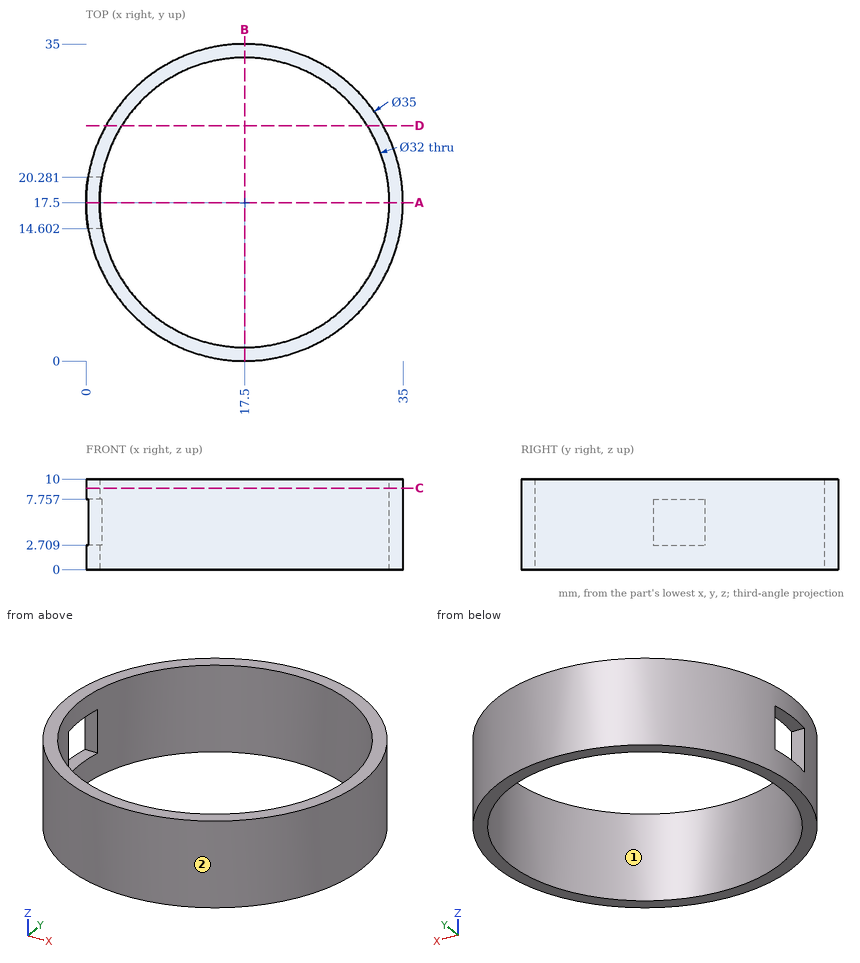
Design review of the part shown in the three views and the two pictorial views. Dimensions are in mm from the part's minimum x, y and z. Give positions to 0.01 mm unless a question says otherwise; leave off trailing zeros. Write each loop counter-clockwise with the first axis right and the second up, starting at its lowest first coordinate (ties: lowest second). Pieces come first, ordered by that corner, then holes. Notation, with made-up numbers: M 70,52 L 116,52 A27 ccw 116,90 Z; hole C 75.25,2.5 d7. An arc over 180 degrees is marked long. One line per question, with ' | ' between items. Start each with the question number.
Item 1: We need section B-B on x = 17.5. Write out the cut boundary in (y, z), plus the area to 3 significant figures.
Item 2: We need section D-D on y = 26. Write out the cut boundary in (x, z) (1 decimal).
Item 3: For pin 1 (3 mm diameter, centred on x = 20.5, y = 4, fed in from +Z); pin 2 (1.5 mm diameter, centred on y = 16.5, z = 2, fed in from -X); pin 3 (3 mm diameter, centred on x = 12, z = 3.5, fed in from +Y); pin 4 (4 mm diameter, centred on y = 26.5, z = 7, fed in from -X), all flat-tipped, find the tip position at first contact; note any pin that passes through.
Item 4: Wall thickness on line 1 (Y direction, x = 17.5, z = 2.5); line 2 (X direction, y = 25, z = 0.5) (1 decimal): over which ranges is each line inside the solid? List them lowest first. Write a range as from..to.
Item 5: We need section C-C on z = 9. Write out the cut boundary in (x, y).
Item 6: Draft analysis for pull direction Y (two halves, no side actions). For the marked faces 1 and 2, state which applies: released by +Y, released by -Y, zero draft, split by the parting line, or undercut.
Item 7: We need section A-A on y = 17.5. Write out the cut boundary in (x, z).
Results found:
1) outline: M 0,0 L 1.5,0 L 1.5,10 L 0,10 Z; M 33.5,0 L 35,0 L 35,10 L 33.5,10 Z | area: 30.0 mm2
2) outline: M 2.2,0 L 3.9,0 L 3.9,10 L 2.2,10 Z; M 31.1,0 L 32.8,0 L 32.8,10 L 31.1,10 Z
3) pin 1: passes through | pin 2: stops at x = 0 | pin 3: stops at y = 34.54 | pin 4: stops at x = 1.46
4) line 1: y = 0..1.5, 33.5..35 | line 2: x = 1.7..3.4, 31.6..33.3
5) outline: C 17.5,17.5 d35; hole C 17.5,17.5 d32
6) face 1: undercut | face 2: split by the parting line
7) outline: M 0,0 L 1.5,0 L 1.5,2.71 L 0,2.71 Z; M 0,7.76 L 1.5,7.76 L 1.5,10 L 0,10 Z; M 33.5,0 L 35,0 L 35,10 L 33.5,10 Z
